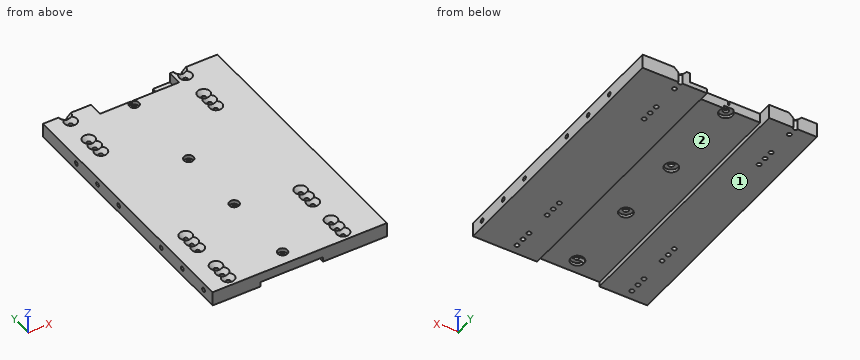
```python
from build123d import *

# Parameters (mm, degrees)
PAD_DEPTH           = 10
SKETCH001_R         = 7
POCKET_DEPTH        = 3
HOLE_D              = 5.8
HOLE_DEPTH          = 25
HOLE_CBORE_D        = 10.1
HOLE_CBORE_DEPTH    = 4.1
SKETCH033_W         = 67
SKETCH033_H         = 280
SKETCH033_W_2       = 50
PAD009_DEPTH        = 5
SKETCH034_R         = 2.25
HOLE009_DEPTH       = 182.501
HOLE015_D           = 4.5
HOLE015_DEPTH       = 25
HOLE015_CSINK_D     = 13
HOLE015_CSINK_ANGLE = 90


with BuildPart() as part:
    # Sketch → Pad (new body)
    with BuildSketch(Plane.XY):
        Polygon((-82.5, 265), (-82.5, -15), (99.5, -15), (99.5, 265), (50, 265), (50, 250), (-32.5, 250), (-32.5, 265), align=None)
    extrude(amount=PAD_DEPTH)

    # Sketch001 → Pocket (cut)
    with BuildSketch(Plane.XY):
        Circle(SKETCH001_R)
        with Locations((0, 80)):
            Circle(SKETCH001_R)
        with Locations((0, 155)):
            Circle(SKETCH001_R)
        with Locations((0, 245)):
            Circle(SKETCH001_R)
    extrude(amount=POCKET_DEPTH, mode=Mode.SUBTRACT)

    # Hole
    with Locations(Plane.XY.offset(10)):
        with Locations((0, 0), (0, 80), (0, 155), (0, 245)):
            CounterBoreHole(HOLE_D / 2, HOLE_CBORE_D / 2, HOLE_CBORE_DEPTH, depth=HOLE_DEPTH)

    # Sketch033 → Pad009 (join)
    with BuildSketch(Plane.XY):
        with Locations((66, 125)):
            Rectangle(SKETCH033_W, SKETCH033_H)
        with Locations((-57.5, 125)):
            Rectangle(SKETCH033_W_2, SKETCH033_H)
    extrude(amount=-PAD009_DEPTH)

    # Sketch034 → Hole009 (cut, through all)
    with BuildSketch(Plane.YZ.offset(100)):
        with Locations((0, 2.5)):
            Circle(SKETCH034_R)
        with Locations((35, 2.5)):
            Circle(SKETCH034_R)
        with Locations((70, 2.5)):
            Circle(SKETCH034_R)
        with Locations((140, 2.5)):
            Circle(SKETCH034_R)
        with Locations((175, 2.5)):
            Circle(SKETCH034_R)
        with Locations((210, 2.5)):
            Circle(SKETCH034_R)
    extrude(amount=-HOLE009_DEPTH, mode=Mode.SUBTRACT)

    # Hole015
    with Locations(Plane.XY.offset(10)):
        with Locations((-60, 255), (-60, 205), (60, 255), (60, 205), (60, 45), (60, -5), (-60, -5), (-60, 45), (60, 55), (60, 5), (-60, 5), (-60, 55), (60, 65), (60, 15), (-60, 15), (-60, 65), (-60, 265), (-60, 215), (60, 265), (60, 215), (-60, 275), (-60, 225), (60, 275), (60, 225)):
            CounterSinkHole(HOLE015_D / 2, HOLE015_CSINK_D / 2, depth=HOLE015_DEPTH, counter_sink_angle=HOLE015_CSINK_ANGLE)


solid = part.part
```
Here's how the part is built. I have some questions about the finished solid (model axes, mm). Face numbers are marked on the shaded views. A direction names the side the tool comes from. Give positions to 0.01 mm unless a question says otherwise; leave off trailing zeros. Loops run counter-clockwise (first coordinate to the right, second up) from the corner with the lowest first, then second, coordinate; pieces in that order, holes last. Notation, with made-up numbers: (57.25, 44.25) -> (110.25, 44.25) arc R16 ccw to (110.25, 68.25) -> close; hole circle Ø5 at (68, -25.75). An arc over 180 degrees is marked (long way). Use one line per item in the form item = value. Start each with the question number.
1) Imagine slicing it at B-B (x = -70). Please give me the cut outline in (y, z).
2) Which directions (+Z, -Z, +X, -X, +Y, -Y) give clear straight access to the entire face, cutting with the end or side of a thin tool? Please do the marked faces 1 and 2.
3) Please list where these lines run through material, in increasing order: line 1 along X through (y, z) = (15, 0.75); line 2 along Y through (x, z) = (0, 5.15); line 3 along X through (y, z) = (243.5, -0.5).
4) For P1, Ø1, axis at x = -28.5, z = 3, coming from the +Y side; P2, Ø2.5, axis at x = 2.5, y = 4.5, coming from the -Z side; P3, Ø6, axis at x = 60, y = 225, coming from the +Z side, each with a flat end and sliding along its axis, tell me the tip position at first contact or that it passes through.
5) Imagine slicing it at A-A (y = 80). Please give me the cut outline in (x, z).
Check values:
q1.outline = (-15, -5) -> (265, -5) -> (265, 10) -> (-15, 10) -> close; hole circle Ø4.5 at (0, 2.5); hole circle Ø4.5 at (35, 2.5); hole circle Ø4.5 at (70, 2.5); hole circle Ø4.5 at (140, 2.5); hole circle Ø4.5 at (175, 2.5); hole circle Ø4.5 at (210, 2.5)
q2.face_1 = -Z, +X, -X, +Y, -Y
q2.face_2 = -Z, +Y, -Y
q3.line_1 = -82.5 to -62.25, -57.75 to 57.75, 62.25 to 99.5
q3.line_2 = -15 to -2.9, 2.9 to 77.1, 82.9 to 152.1, 157.9 to 242.1, 247.9 to 250
q3.line_3 = -82.5 to -32.5, 32.5 to 99.5
q4.P1 = 250
q4.P2 = 3
q4.P3 = 6.5
q5.outline = (-82.5, -5) -> (-32.5, -5) -> (-32.5, 0) -> (-7, 0) -> (-7, 3) -> (-2.9, 3) -> (-2.9, 5.9) -> (-5.05, 5.9) -> (-5.05, 10) -> (-82.5, 10) -> close; (2.9, 3) -> (7, 3) -> (7, 0) -> (32.5, 0) -> (32.5, -5) -> (99.5, -5) -> (99.5, 10) -> (5.05, 10) -> (5.05, 5.9) -> (2.9, 5.9) -> close
